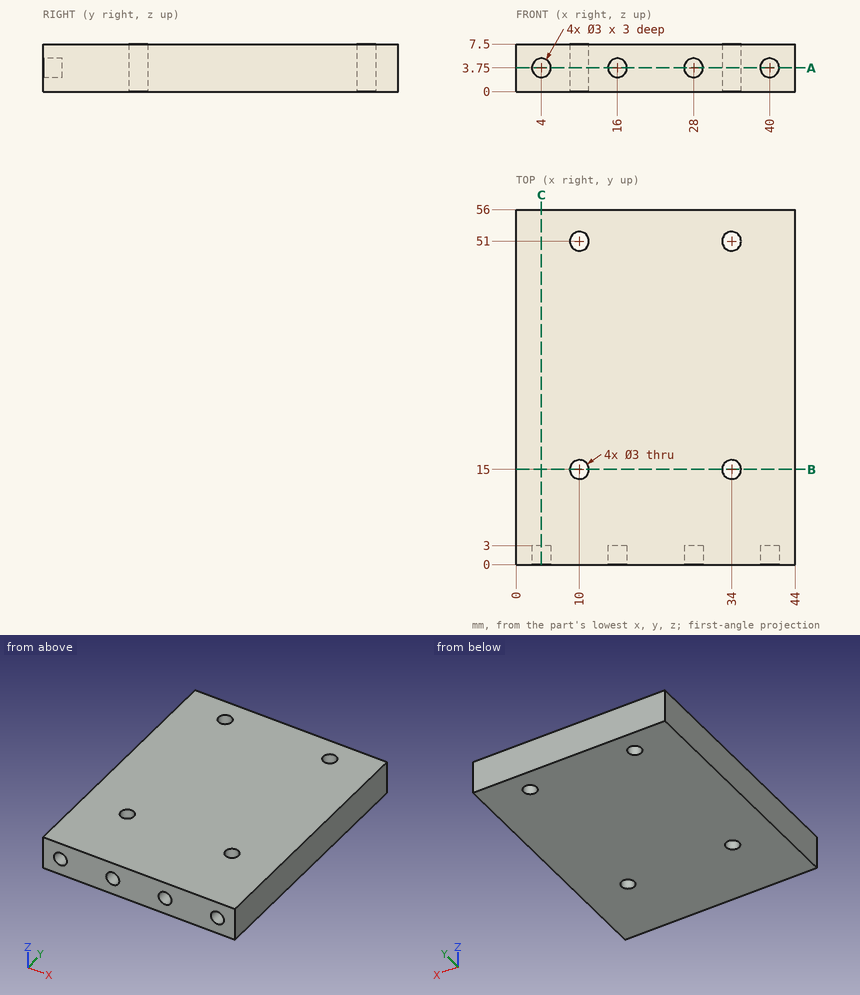
Drawing for the job (mm, zero at the part's lowest x, y, z). Round coordinates to 2 decimals unless told otherwise and drop trailing zeros. Write each loop counter-clockwise with the first axis right and the second up, starting at its lowest first coordinate (ties: lowest second). Pieces come first, ordered by that corner, then holes. Notation, with made-up numbers: M 75,-30 L 99,-30 A24 cw 99,6 Z; hole C 41,67 d3. An arc over 180 degrees is marked long. Answer in a Markdown table with one row per item.
1. Saw through at B-B (y = 15). List the corners of the cut face in (x, z).
Geometry check:
| item | result |
|---|---|
| outline | M 0,0 L 8.5,0 L 8.5,7.5 L 0,7.5 Z; M 11.5,0 L 32.5,0 L 32.5,7.5 L 11.5,7.5 Z; M 35.5,0 L 44,0 L 44,7.5 L 35.5,7.5 Z |
2. Probe L1, parallel to X at y = 0.9, z = 3.75; L2, parallel to Y at x = 34, z = 5.25; L3, parallel to X at y = 14, z = 6. List the from-to ranges inside material, lowest first. Write a range as [from, to].
Geometry check:
| item | result |
|---|---|
| L1 | [0, 2.5], [5.5, 14.5], [17.5, 26.5], [29.5, 38.5], [41.5, 44] |
| L2 | [0, 13.5], [16.5, 49.5], [52.5, 56] |
| L3 | [0, 8.88], [11.12, 32.88], [35.12, 44] |
3. Flat gauge pins, fed straight in: P1, Ø2.5, axis at x = 28, z = 3.75, coming from the -Y side; P2, Ø2.5, axis at x = 34, y = 51, coming from the +Z side. Where does each tip first touch, or does it go through?
Geometry check:
| item | result |
|---|---|
| P1 | y = 3 |
| P2 | through |
4. Saw through at A-A (z = 3.75). List the corners of the cut face in (x, y), and give its area (3 significant figures).
Geometry check:
| item | result |
|---|---|
| outline | M 0,0 L 2.5,0 L 2.5,3 L 5.5,3 L 5.5,0 L 14.5,0 L 14.5,3 L 17.5,3 L 17.5,0 L 26.5,0 L 26.5,3 L 29.5,3 L 29.5,0 L 38.5,0 L 38.5,3 L 41.5,3 L 41.5,0 L 44,0 L 44,56 L 0,56 Z; hole C 10,15 d3; hole C 10,51 d3; hole C 34,15 d3; hole C 34,51 d3 |
| area | 2,400 mm2 |
5. Saw through at C-C (x = 4). List the corners of the cut face in (y, z).
Geometry check:
| item | result |
|---|---|
| outline | M 0,0 L 56,0 L 56,7.5 L 0,7.5 L 0,5.25 L 3,5.25 L 3,2.25 L 0,2.25 Z |
